Geometry check sheet. Reference: the model listing, model coordinates, mm. A direction names the side the tool comes from. Round coordinates to 2 decimals unless told otherwise and drop trailing zeros. Write each loop counter-clockwise with the first axis right and the second up, starting at its lowest first coordinate (ties: lowest second). Pieces come first, ordered by that corner, then holes. Notation, with made-up numbers: (65, 0.25) -> (100, 0.25) arc R20 cw to (100, 14.25) -> close; hole circle Ø3 at (-18.75, 35). An arc over 180 degrees is marked (long way). Return JSON: item names as keys, results as strings. Group by question number.
from build123d import *

# Parameters (mm, degrees)
ESQUISSE3_W                   = 53.75
ESQUISSE3_H                   = 73.333333334
BOSS_EXTRU_2_DEPTH            = 6.35
CONG_6_R                      = 20
CONG_7_R                      = 15
ESQUISSE4_R                   = 2.25
ENL_V_MAT_EXTRU_2_DEPTH       = 6.35
SYM_TRIE2_COPY_1_SKETCH_R     = 2.25
SYM_TRIE2_COPY_1_DEPTH        = 6.35
DIAM_TRE_DU_PER_AGE_4_0_4_1_D = 4
ESQUISSE9_OUTSIDE_W           = 257.77
ESQUISSE9_OUTSIDE_H           = 212.77
ENL_V_MAT_EXTRU_3_DEPTH       = 130.491560966
ESQUISSE10_R                  = 2.25
ENL_V_MAT_EXTRU_4_DEPTH       = 130.491560966


with BuildPart() as part:
    # Esquisse3 → Boss.-Extru.2 (new body)
    with BuildSketch(Plane.XY):
        Polygon((-54.672450369, 55), (54.672450369, 55), (71.992958445, 85), (107.5, 64.5), (77.5, 12.538475773), (77.5, -12.538475773), (107.5, -64.5), (71.992958445, -85), (54.672450369, -55), (-54.672450369, -55), (-71.992958445, -85), (-107.5, -64.5), (-77.5, -12.538475773), (-77.5, 12.538475773), (-107.5, 64.5), (-71.992958445, 85), align=None)
        Rectangle(ESQUISSE3_W, ESQUISSE3_H, mode=Mode.SUBTRACT)
    extrude(amount=-BOSS_EXTRU_2_DEPTH)

    # Congé6
    cong_6_edges = [part.edges().sort_by_distance(p)[0] for p in [
        (-54.672450369, 55, -3.175),
        (54.672450369, 55, -3.175),
        (77.5, 12.538475773, -3.175),
        (77.5, -12.538475773, -3.175),
        (54.672450369, -55, -3.175),
        (-54.672450369, -55, -3.175),
        (-77.5, -12.538475773, -3.175),
        (-77.5, 12.538475773, -3.175),
        (-26.875, -36.666666667, -3.175),
        (-26.875, 36.666666667, -3.175),
        (26.875, 36.666666667, -3.175),
        (26.875, -36.666666667, -3.175),
    ]]
    fillet(cong_6_edges, radius=CONG_6_R)

    # Congé7
    cong_7_edges = [part.edges().sort_by_distance(p)[0] for p in [
        (71.992958445, 85, -3.175),
        (107.5, 64.5, -3.175),
        (107.5, -64.5, -3.175),
        (71.992958445, -85, -3.175),
        (-71.992958445, -85, -3.175),
        (-107.5, -64.5, -3.175),
        (-107.5, 64.5, -3.175),
        (-71.992958445, 85, -3.175),
    ]]
    fillet(cong_7_edges, radius=CONG_7_R)

    # Esquisse4 → Enlèv. mat.-Extru.2 (cut)
    with BuildSketch(Plane.XY):
        with Locations((-56.291352203, 26.80402023)):
            Circle(ESQUISSE4_R)
        with Locations((-64.951606241, 21.80402023)):
            Circle(ESQUISSE4_R)
        with Locations((-89.201606241, 63.806252313)):
            Circle(ESQUISSE4_R)
        with Locations((-80.541352203, 68.806252313)):
            Circle(ESQUISSE4_R)
        Polygon((-53.283116293, 32.293602792), (-74.283116293, 68.666669751), (-92.209842152, 58.316669751), (-71.209842152, 21.943602792), align=None)
        with BuildLine():
            Line((-51.695036381, 4.342967697), (-54.695036381, 9.53912012))
            ThreePointArc((-54.695036381, 9.53912012), (-53.871479222, 12.612677278), (-50.797922064, 11.78912012))
            Line((-50.797922064, 11.78912012), (-47.797922064, 6.592967697))
            ThreePointArc((-47.797922064, 6.592967697), (-48.621479222, 3.519410539), (-51.695036381, 4.342967697))
        make_face()
    enl_v_mat_extru_2 = extrude(amount=-ENL_V_MAT_EXTRU_2_DEPTH, mode=Mode.SUBTRACT)

    # Symétrie1: Enlèv. mat.-Extru.2 across plane
    add(enl_v_mat_extru_2.mirror(Plane.ZX), mode=Mode.SUBTRACT)

    # Symétrie2: Enlèv. mat.-Extru.2 across plane
    add(enl_v_mat_extru_2.mirror(Plane(origin=(0, 0, 0), x_dir=(0, 0, 1), z_dir=(1, 0, 0))), mode=Mode.SUBTRACT)

    # Symétrie2 copy 1 sketch → Symétrie2 copy 1 (cut)
    with BuildSketch(Plane(origin=(0, 0, 0), x_dir=(-1, 0, 0), z_dir=(0, 0, 1))):
        with Locations((-56.291352203, 26.80402023)):
            Circle(SYM_TRIE2_COPY_1_SKETCH_R)
        with Locations((-64.951606241, 21.80402023)):
            Circle(SYM_TRIE2_COPY_1_SKETCH_R)
        with Locations((-89.201606241, 63.806252313)):
            Circle(SYM_TRIE2_COPY_1_SKETCH_R)
        with Locations((-80.541352203, 68.806252313)):
            Circle(SYM_TRIE2_COPY_1_SKETCH_R)
        Polygon((-53.283116293, 32.293602792), (-74.283116293, 68.666669751), (-92.209842152, 58.316669751), (-71.209842152, 21.943602792), align=None)
        with BuildLine():
            Line((-51.695036381, 4.342967697), (-54.695036381, 9.53912012))
            ThreePointArc((-54.695036381, 9.53912012), (-53.871479222, 12.612677278), (-50.797922064, 11.78912012))
            Line((-50.797922064, 11.78912012), (-47.797922064, 6.592967697))
            ThreePointArc((-47.797922064, 6.592967697), (-48.621479222, 3.519410539), (-51.695036381, 4.342967697))
        make_face()
    extrude(amount=-SYM_TRIE2_COPY_1_DEPTH, mode=Mode.SUBTRACT)

    # Diamètre du perçage Ø4.0 (4)1 (through all)
    with Locations(Plane.XY):
        with Locations((33, 48), (-33, 48), (-33, -48), (33, -48)):
            Hole(DIAM_TRE_DU_PER_AGE_4_0_4_1_D / 2)

    # Esquisse9 outside → Enlèv. mat.-Extru.3 (cut, through all)
    with BuildSketch(Plane.XY):
        Rectangle(ESQUISSE9_OUTSIDE_W, ESQUISSE9_OUTSIDE_H)
        with BuildLine():
            Line((-65.608946312, 73.674704124), (-92.209842152, 58.316669751))
            Line((-92.209842152, 58.316669751), (-82.209842152, 40.996161675))
            Line((-82.209842152, 40.996161675), (-91, 35.921161675))
            Line((-91, 35.921161675), (-100, 51.509618943))
            ThreePointArc((-100, 51.509618943), (-101.498506338, 62.89190462), (-94.509618943, 72))
            Line((-94.509618943, 72), (-84.983339502, 77.5))
            ThreePointArc((-84.983339502, 77.5), (-74.577818709, 79.225526966), (-65.608946312, 73.674704124))
        make_face(mode=Mode.SUBTRACT)
    extrude(amount=-ENL_V_MAT_EXTRU_3_DEPTH, mode=Mode.SUBTRACT)

    # Esquisse10 → Enlèv. mat.-Extru.4 (cut, through all)
    with BuildSketch(Plane.XY):
        with Locations((-91.104921076, 46.252890309)):
            Circle(ESQUISSE10_R)
        with Locations((-72.574022775, 74.849567776)):
            Circle(ESQUISSE10_R)
    extrude(amount=-ENL_V_MAT_EXTRU_4_DEPTH, mode=Mode.SUBTRACT)


solid = part.part
1) Tool access check on faces 1 (the face through (-87.28, 49.78, -3.13)), 2 (the face through (-74.82, 74.95, -3.13)). Record the directions out of +Z, -Z, +X, -X, +Y, -Y that give a thin tool (end or side, any length) a straight path to the whole face; none if there is none.
2) Material ranges on probe 1 along Y at (x, z) = (-87.5, -3); probe 2 along Y at (x, z) = (-78.5, -1.5); probe 3 along X at (y, z) = (69, -6), recorded low to high. Write a range as [from, to].
3) Sectioned sample at D-D on y = 53.5. Enter the section's corners in (x, z).
4) Sectioned sample at C-C on x = -86. Enter the section's corners in (y, z), and give its area (3 significant figures).
5) Sectioned sample at B-B on z = -1.5. Enter the section's corners in (x, y).
6) Mould release check, pull along Y, two halves, no side actions. Record for faces 3 (the face through (-101.455, 63.051, -3.219)), 4 (the face through (-89.813, 74.712, -3.131)), 5 (the face through (-92.89, 44.88, -3.13)), 6 (the face through (-82.79, 68.91, -3.13)): +Y half, -Y half, draft (parallel to the pull), parting line (faces both ways), or undercut.
7) Sectioned sample at A-A on x = -71. Enter the section's corners in (y, z), and give its area (3 significant figures).
Evaluation:
{
 "1": {"face 1": "+Z, -Z, +X", "face 2": "+Z, -Z"},
 "2": {"probe 1": "y = [37.94, 50.16], [61.04, 62.33], [65.28, 76.05]", "probe 2": "y = [66.23, 67.86], [69.75, 79.48]", "probe 3": "x = [-98.2, -82.78], [-78.3, -73.71]"},
 "3": {"outline": "(-100.96, -6.35) -> (-89.43, -6.35) -> (-89.43, 0) -> (-100.96, 0) -> close"},
 "4": {"outline": "(38.81, -6.35) -> (47.56, -6.35) -> (47.56, 0) -> (38.81, 0) -> close; (61.9, -6.35) -> (76.91, -6.35) -> (76.91, 0) -> (61.9, 0) -> close", "area": "151 mm2"},
 "5": {"outline": "(-100, 51.51) -> (-91, 35.92) -> (-82.21, 41) -> (-92.21, 58.32) -> (-65.61, 73.67) arc R15 ccw to (-84.98, 77.5) -> (-94.51, 72) arc R15 ccw to start; hole circle Ø4.5 at (-91.1, 46.25); hole circle Ø4.5 at (-89.2, 63.81); hole circle Ø4.5 at (-80.54, 68.81); hole circle Ø4.5 at (-72.57, 74.85)"},
 "6": {"face 3": "parting line", "face 4": "+Y half", "face 5": "undercut", "face 6": "undercut"},
 "7": {"outline": "(70.56, -6.35) -> (73.24, -6.35) -> (73.24, 0) -> (70.56, 0) -> close; (76.46, -6.35) -> (78.04, -6.35) -> (78.04, 0) -> (76.46, 0) -> close", "area": "27.0 mm2"}
}
